Source: CAD feature listing. Evaluate the final solid. Frame: model axes, mm. Face numbers are marked on the shaded views. A direction names the side the tool comes from. Round coordinates to 2 decimals unless told otherwise and drop trailing zeros. Order: outer loops, then holes, each group sorted by start corner. A loop starts at its lowest first (then second) coordinate and runs counter-clockwise, first axis right, second up. Notation, with made-up numbers: (-27.5, -38) - (7.5, -38) arc R21 cw to (7.5, -1) - close; hole circle Ø9 at (-8, 78). An arc over 180 degrees is marked (long way). Return JSON: item names as keys, results as strings. Group by question number.
1) Section D-D, the plane y = -12. Return loops of the section in (x, z).
2) Section B-B, the plane x = -30.5. Return loops of the section in (y, z).
3) Contact query for flat-ended pins moving along their axis: P1, Ø3, axis at x = -10, z = 28.5, coming from the -Y side; P2, Ø6, axis at y = -44.5, z = 36.5, coming from the +X side; P3, Ø14, axis at y = -35, z = 3, coming from the -X side; P4, Ø10, axis at y = -45.5, z = 17.5, coming from the -X side. Output: stop coordinate, or through.
4) Ray query, line 1 (X direction, y = -2, z = 22.5); line 2 (Y direction, x = -22.5, z = 2). Return the intervals inside material, ascending. Write a range as from..to.
5) Access query for the marked faces 1, 2, 3, 4 and 5. Directions: +Z, -Z, +X, -X, +Y, -Y. A direction counts if a zero-diameter tool reaches every point of the face in a straight line with its end or side. Return the directions, or none.
6) Section A-A, the plane y = -30.5. Return loops of the section in (x, z), plus the area to 3 significant figures.
7) Mould query, pull axis X, two halves, no side actions, for the marked faces 6, 7 and 8. Classes: pulls with the +X half, pulls with the -X half, needs draft (parallel to the pull), parting line crosses it, or undercut.
8) Section C-C, the plane z = 22.5. Return loops of the section in (x, y), plus the area to 3 significant figures.
```python
from build123d import *

# Parameters (mm, degrees)
BOSS_EXTRU_1_DEPTH      = 45
ENL_V_MAT_EXTRU_1_REACH = 55
ESQUISSE2_R             = 5
ENL_V_START             = -12.5
ESQUISSE3_W             = 37.334250657
ESQUISSE3_H             = 36.0198364
ENL_V_MAT_EXTRU_2_DEPTH = 20
ESQUISSE4_R             = 10
BOSS_EXTRU_2_DEPTH      = 4
ENL_V_MAT_EXTRU_3_REACH = 59
ESQUISSE5_R             = 5


with BuildPart() as part:
    # Esquisse1 → Boss.-Extru.1 (new body)
    with BuildSketch(Plane.XY):
        Polygon((-53, 0), (0, 0), (0, -53), (-8, -53), (-8, -35.552659183), (-15, -35.552659183), (-15, -40), (-19, -40), (-19, -21), (-15, -21), (-15, -25.447340817), (-8, -25.447340817), (-8, -8), (-25.447340817, -8), (-25.447340817, -15), (-21, -15), (-21, -19), (-40, -19), (-40, -15), (-35.552659183, -15), (-35.552659183, -8), (-53, -8), align=None)
    extrude(amount=BOSS_EXTRU_1_DEPTH)

    # Esquisse2 → Enlèv. mat.-Extru.1 (cut, up to next)
    with BuildSketch(Plane(origin=(0, 0, 0), x_dir=(0, 0, -1), z_dir=(1, 0, 0)), mode=Mode.PRIVATE) as enl_v_mat_extru_1_sk1:
        with Locations((-22.5, -30.5)):
            Circle(ESQUISSE2_R)
    enl_v_mat_extru_1_tool1 = extrude(enl_v_mat_extru_1_sk1.sketch, amount=-ENL_V_MAT_EXTRU_1_REACH, mode=Mode.PRIVATE) & part.part
    add(enl_v_mat_extru_1_tool1.solids().sort_by_distance((0, -30.5, 22.5))[0], mode=Mode.SUBTRACT)

    # Esquisse3 → Enlèv. mat.-Extru.2 (cut)
    with BuildSketch(Plane(origin=(0, 0, 0), x_dir=(-1, 0, 0), z_dir=(0, 0, -1)).offset(ENL_V_START)):
        with Locations((26.667125329, -26.0099182)):
            Rectangle(ESQUISSE3_W, ESQUISSE3_H)
    extrude(amount=-ENL_V_MAT_EXTRU_2_DEPTH, mode=Mode.SUBTRACT)

    # Esquisse4 → Boss.-Extru.2 (add)
    with BuildSketch(Plane(origin=(0, 0, 0), x_dir=(1, 0, 0), z_dir=(0, 1, 0))):
        with Locations((-30.5, -22.5)):
            Circle(ESQUISSE4_R)
    extrude(amount=BOSS_EXTRU_2_DEPTH)

    # Esquisse5 → Enlèv. mat.-Extru.3 (cut, up to next)
    with BuildSketch(Plane(origin=(0, 4, 0), x_dir=(1, 0, 0), z_dir=(0, 1, 0)), mode=Mode.PRIVATE) as enl_v_mat_extru_3_sk1:
        with Locations((-30.5, -22.5)):
            Circle(ESQUISSE5_R)
    enl_v_mat_extru_3_tool1 = extrude(enl_v_mat_extru_3_sk1.sketch, amount=-ENL_V_MAT_EXTRU_3_REACH, mode=Mode.PRIVATE) & part.part
    add(enl_v_mat_extru_3_tool1.solids().sort_by_distance((-30.5, 4, 22.5))[0], mode=Mode.SUBTRACT)


solid = part.part
```
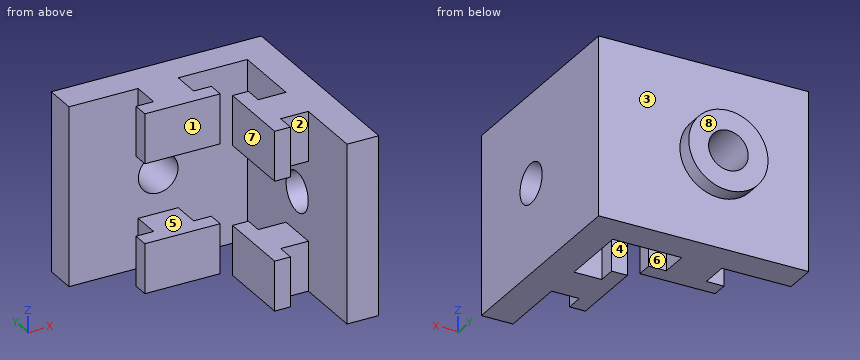
Geometry check:
{
 "1": {"outline": "(-35.55, 0) - (-25.45, 0) - (-25.45, 12.5) - (-35.55, 12.5) - close; (-35.55, 32.5) - (-25.45, 32.5) - (-25.45, 45) - (-35.55, 45) - close; (-8, 0) - (0, 0) - (0, 45) - (-8, 45) - close"},
 "2": {"outline": "(-19, 0) - (0, 0) - (0, 12.5) - (4, 12.5) - (4, 17.5) - (-8, 17.5) - (-8, 12.5) - (-19, 12.5) - close; (-19, 32.5) - (-8, 32.5) - (-8, 27.5) - (4, 27.5) - (4, 32.5) - (0, 32.5) - (0, 45) - (-19, 45) - close"},
 "3": {"P1": "y = -8", "P2": "x = 0", "P3": "x = -19", "P4": "x = -8"},
 "4": {"line 1": "-53..-35.5, -25.5..0", "line 2": "-19..-15, -8..0"},
 "5": {"face 1": "+Z, -Z, -X, -Y", "face 2": "+Z, -Z, -Y", "face 3": "+Y", "face 4": "+Z, -Z, -X", "face 5": "-X, -Y"},
 "6": {"outline": "(-19, 0) - (0, 0) - (0, 17.5) - (-8, 17.5) - (-8, 12.5) - (-19, 12.5) - close; (-19, 32.5) - (-8, 32.5) - (-8, 27.5) - (0, 27.5) - (0, 45) - (-19, 45) - close", "area": "555 mm2"},
 "7": {"face 6": "undercut", "face 7": "pulls with the -X half", "face 8": "needs draft"},
 "8": {"outline": "(-53, -8) - (-35.5, -8) - (-35.5, 4) - (-40.5, 4) - (-40.5, 0) - (-53, 0) - close; (-25.5, -8) - (-8, -8) - (-8, -25.5) - (0, -25.5) - (0, 0) - (-20.5, 0) - (-20.5, 4) - (-25.5, 4) - close; (-8, -53) - (0, -53) - (0, -35.5) - (-8, -35.5) - close", "area": "664 mm2"}
}
